The figure shows three views and two pictorial views of one solid part (mm, origin at its lowest corner). Answer the questions. Coordinates: 2 decimals unless noted, no trailing zeros. Loops run counter-clockwise (first coordinate to the right, second up) from the corner with the lowest first, then second, coordinate; pieces in that order, holes last. Notation, with made-up numbers: (-26.5, 17.5) - (22.5, 17.5) arc R14 cw to (22.5, 29.5) - close; hole circle Ø1 at (-39, 12). An arc over 180 degrees is marked (long way). One line per question, with ' | ' between items.
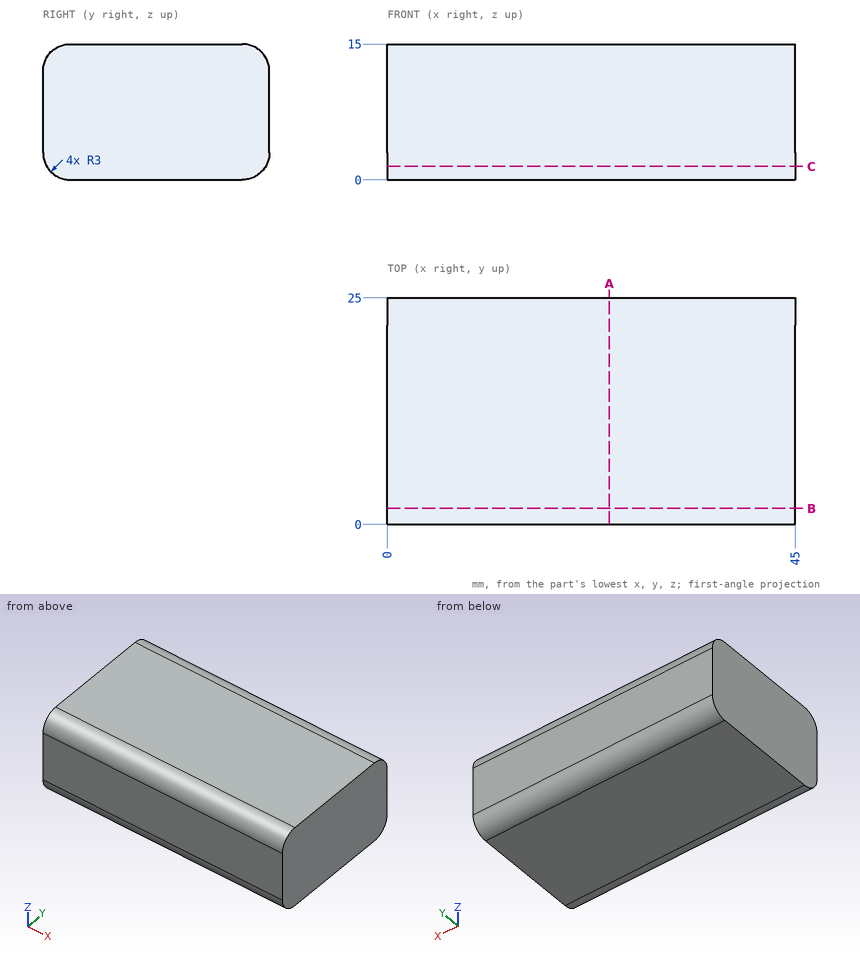
Item 1: Find section B-B, the plane y = 1.75. Write down the section's boundary in (x, z).
Taken from the geometry:
outline: (0, 0.27) - (45, 0.27) - (45, 14.73) - (0, 14.73) - close
Item 2: Find section A-A, the plane x = 24.5. Write down the section's boundary in (y, z), plus the area to 3 significant figures.
Taken from the geometry:
outline: (0, 3) arc R3 ccw to (3, 0) - (22, 0) arc R3 ccw to (25, 3) - (25, 12) arc R3 ccw to (22, 15) - (3, 15) arc R3 ccw to (0, 12) - close | area: 367 mm2
Item 3: Find section C-C, the plane z = 1.5. Write down the section's boundary in (x, y).
Taken from the geometry:
outline: (0, 0.4) - (45, 0.4) - (45, 24.6) - (0, 24.6) - close
Item 4: Find the intervals of material crossed by line 1 (Y direction, x = 8, z = 2.75); line 2 (Y direction, x = 8, z = 13); line 3 (Z direction, x = 23, y = 1.5), in increasing order. Write a range as [from, to].
Taken from the geometry:
line 1: y = [0.01, 24.99] | line 2: y = [0.17, 24.83] | line 3: z = [0.4, 14.6]
